Can you work these out from the model? Positions are in its coordinate system, mm. A direction names the side the tool comes from. Coordinates: 2 decimals unless noted, no trailing zeros.
```python
from build123d import *

# Parameters (mm, degrees)
BOSS_EXTRUDE1_DEPTH = 50
SKETCH2_R           = 200
CUT_EXTRUDE1_DEPTH  = 12.5
SKETCH3_R           = 100
BOSS_EXTRUDE2_DEPTH = 12.5
FILLET1_R           = 10
FILLET8_R           = 10
FILLET10_R          = 10
FILLET11_R          = 10
SKETCH4_R           = 6
BOSS_EXTRUDE3_DEPTH = 36
CIRPATTERN1_COUNT   = 3


with BuildPart() as part:
    # Sketch1 → Boss-Extrude1 (new body)
    with BuildSketch(Plane(origin=(0, 0, 0), x_dir=(1, 0, 0), z_dir=(0, 1, 0))):
        with BuildLine():
            Line((177.17937854, -160.029588814), (223.117233569, -186.551821781))
            Line((223.117233569, -186.551821781), (235.617233569, -164.901186686))
            Line((235.617233569, -164.901186686), (193.127700242, -140.369843182))
            ThreePointArc((193.127700242, -140.369843182), (206.764361308, -119.37545966), (218.127700242, -97.068572993))
            Line((218.127700242, -97.068572993), (260.617233569, -121.599916497))
            Line((260.617233569, -121.599916497), (273.117233569, -99.949281403))
            Line((273.117233569, -99.949281403), (227.17937854, -73.427048436))
            ThreePointArc((227.17937854, -73.427048436), (206.764361308, 119.37545966), (50, 233.45663725))
            Line((50, 233.45663725), (50, 286.501103184))
            Line((50, 286.501103184), (25, 286.501103184))
            Line((25, 286.501103184), (25, 237.438416176))
            ThreePointArc((25, 237.438416176), (0, 238.75091932), (-25, 237.438416176))
            Line((-25, 237.438416176), (-25, 286.501103184))
            Line((-25, 286.501103184), (-50, 286.501103184))
            Line((-50, 286.501103184), (-50, 233.45663725))
            ThreePointArc((-50, 233.45663725), (-206.764361308, 119.37545966), (-227.17937854, -73.427048436))
            Line((-227.17937854, -73.427048436), (-273.117233569, -99.949281403))
            Line((-273.117233569, -99.949281403), (-260.617233569, -121.599916497))
            Line((-260.617233569, -121.599916497), (-218.127700242, -97.068572993))
            ThreePointArc((-218.127700242, -97.068572993), (-206.764361308, -119.37545966), (-193.127700242, -140.369843182))
            Line((-193.127700242, -140.369843182), (-235.617233569, -164.901186686))
            Line((-235.617233569, -164.901186686), (-223.117233569, -186.551821781))
            Line((-223.117233569, -186.551821781), (-177.17937854, -160.029588814))
            ThreePointArc((-177.17937854, -160.029588814), (0, -238.75091932), (177.17937854, -160.029588814))
        make_face()
    extrude(amount=BOSS_EXTRUDE1_DEPTH)

    # Sketch2 → Cut-Extrude1 (cut)
    with BuildSketch(Plane(origin=(0, 50, 0), x_dir=(1, 0, 0), z_dir=(0, 1, 0))):
        Circle(SKETCH2_R)
    extrude(amount=-CUT_EXTRUDE1_DEPTH, mode=Mode.SUBTRACT)

    # Sketch3 → Boss-Extrude2 (add)
    with BuildSketch(Plane(origin=(0, 37.5, 0), x_dir=(1, 0, 0), z_dir=(0, 1, 0))):
        Circle(SKETCH3_R)
    extrude(amount=BOSS_EXTRUDE2_DEPTH)

    # Fillet1
    fillet1_edges = [part.edges().sort_by_distance(p)[0] for p in [
        (-37.5, 50, -286.501103184),
        (37.5, 0, -286.501103184),
        (266.867233569, 0, 110.77459895),
        (229.367233569, 0, 175.726504234),
        (-229.367233569, 0, 175.726504234),
        (-266.867233569, 50, 110.77459895),
        (-266.867233569, 0, 110.77459895),
        (-37.5, 0, -286.501103184),
        (-229.367233569, 50, 175.726504234),
        (229.367233569, 50, 175.726504234),
        (266.867233569, 50, 110.77459895),
        (37.5, 50, -286.501103184),
    ]]
    fillet(fillet1_edges, radius=FILLET1_R)

    # Fillet8
    fillet8_edges = [part.edges().sort_by_distance(p)[0] for p in [
        (-100, 50, 0),
    ]]
    fillet(fillet8_edges, radius=FILLET8_R)

    # Fillet10
    fillet10_edges = [part.edges().sort_by_distance(p)[0] for p in [
        (-200, 37.5, 0),
    ]]
    fillet(fillet10_edges, radius=FILLET10_R)

    # Fillet11
    fillet11_edges = [part.edges().sort_by_distance(p)[0] for p in [
        (-200, 50, 0),
    ]]
    fillet(fillet11_edges, radius=FILLET11_R)

    # Sketch4 → Boss-Extrude3 (add, symmetric)
    with BuildSketch(Plane(origin=(0, 0, 0), x_dir=(0, 0, -1), z_dir=(1, 0, 0))):
        with Locations((273.2399867, 25)):
            Circle(SKETCH4_R)
    boss_extrude3 = extrude(amount=BOSS_EXTRUDE3_DEPTH, both=True)

    # CirPattern1: Boss-Extrude3 ×3 about axis
    cirpattern1_axis = Axis((0, 50, 0), (0, -1, 0))
    for i in range(1, CIRPATTERN1_COUNT):
        add(boss_extrude3.rotate(cirpattern1_axis, i * 360 / CIRPATTERN1_COUNT))


solid = part.part
```
1. Thinking about a two-plate mould opening in Z: for faces 1 (the cylindrical face through (208.148, 24.65, -116.947)), 2 (the flat face through (50, 25, -260)), 3 (the cylindrical face through (264.35, 2.85, 109.12)), which applies, pulls with the +Z half, pulls with the -Z half, needs draft (parallel to the pull), parting line crosses it, or undercut?
Completed:
face 1: undercut
face 2: needs draft
face 3: pulls with the +Z half
2. On a 3-axis mill with a long thin cutter (end or side, diameter ignored), from which of +Z, -Z, +X, -X, +Y, -Y can I reach the whole of each face in a straight line? I mean faces 4 (the flat face through (82, 37.5, 82)), 5 (the flat face through (-50, 25, -260)), 6 (the flat face through (199.827, 24.65, 173.105)), 7 (the cylindrical face through (0.35, 24.65, -238.75)). Say none if no direction works.
Completed:
face 4: +Y
face 5: -Z, -X, +Y, -Y
face 6: +Z, +Y, -Y
face 7: +Y, -Y
3. I'm going to push flat-ended pins straight in: pin 1 (4 mm diameter, centred on y = 22.5, z = 52.5, fed in from -X); pin 2 (8 mm diameter, centred on x = -171.5, y = 30, fed in from -Z); pin 3 (14.5 mm diameter, centred on y = 33.5, z = -252.5, fed in from +X). Where does each tip first touch, or does it pass through?
Completed:
pin 1: stops at x = -233.35
pin 2: stops at z = -170.13
pin 3: stops at x = 50
4. Please list where these lines run through material, in increasing order: probe 1 along X at (y, z) = (8, -254); probe 2 along X at (y, z) = (46, 52); probe 3 along Z at (x, y) = (57, 47).
Completed:
probe 1: x = -50 to -25, 25 to 50
probe 2: x = -233.02 to -193.68, -83.07 to 83.07, 193.68 to 233.02
probe 3: z = -231.85 to -193.16, -78.66 to 78.66, 193.16 to 231.85
